The listing builds one solid part. Answer for the finished solid, in the listing's coordinates (mm). Face numbers are marked on the shaded views. A direction names the side the tool comes from. Give positions to 0.01 mm unless a question says otherwise; leave off trailing zeros. Order: outer loops, then holes, each group sorted by start corner. A loop starts at its lowest first (then second) coordinate and runs counter-clockwise, first axis right, second up. Notation, with made-up numbers: (60, -26.75) - (100, -26.75) arc R22 ccw to (100, -9.75) - close; hole circle Ø11 at (59.25, 74). An arc over 180 degrees is marked (long way). Use a Markdown table: item, result. Add a question column.
1) Find section C-C, the plane z = 1. Determine the outline of the cut face in (x, y), plus the area to 3 significant figures.
2) Straight lines are drawn through the part: line 1 (X direction, y = 18.25, z = -6.25); line 2 (Y direction, x = -21, z = 4.5); line 3 (Y direction, x = 14, z = 6.5). For each, find the intervals that lie inside material, in ascending order.
3) Find section D-D, the plane y = 2.25. Determine the outline of the cut face in (x, z).
4) Flat-ended cylindrical pins translate along their axes: pin 1 (5 mm diameter, centred on x = -20.5, z = 0.5, fed in from +Y); pin 2 (2 mm diameter, centred on x = 14.5, z = -3.5, fed in from +Y). Find the tip coordinate at first contact, or state that the pin passes through.
5) The mould has two halves that part along X. Classify the marked faces 1, 2 and 3: released by +X, released by -X, zero draft, split by the parting line, or undercut.
6) For the marked faces 4 and 5, determine the directions among +Z, -Z, +X, -X, +Y, -Y from which every point of the face is accessible in a straight line to the end or side of a thin tool.
7) Find section A-A, the plane y = 12.25. Determine the outline of the cut face in (x, z), plus the area to 3 significant figures.
8) Find section B-B, the plane x = -7. Determine the outline of the cut face in (y, z).
from build123d import *

# Parameters (mm, degrees)
SKETCH1_W           = 52
SKETCH1_H           = 18
BOSS_EXTRUDE1_DEPTH = 25.5
SKETCH2_W           = 46.1
SKETCH2_H           = 14.1
CUT_EXTRUDE1_DEPTH  = 2.5
SKETCH4_W           = 40
SKETCH4_H           = 18
CUT_EXTRUDE2_DEPTH  = 22.5
SKETCH5_W           = 25
SKETCH5_H           = 10
CUT_EXTRUDE3_DEPTH  = 4
FILLET1_R           = 2
FILLET2_R           = 2


with BuildPart() as part:
    # Sketch1 → Boss-Extrude1 (new body)
    with BuildSketch(Plane(origin=(0, 0, 0), x_dir=(1, 0, 0), z_dir=(0, 1, 0))):
        Rectangle(SKETCH1_W, SKETCH1_H)
    extrude(amount=BOSS_EXTRUDE1_DEPTH)

    # Sketch2 → Cut-Extrude1 (cut)
    with BuildSketch(Plane(origin=(0, 25.5, 0), x_dir=(1, 0, 0), z_dir=(0, 1, 0))):
        Rectangle(SKETCH2_W, SKETCH2_H)
    extrude(amount=-CUT_EXTRUDE1_DEPTH, mode=Mode.SUBTRACT)

    # Sketch4 → Cut-Extrude2 (cut)
    with BuildSketch(Plane(origin=(0, 25.5, 0), x_dir=(1, 0, 0), z_dir=(0, 1, 0))):
        Rectangle(SKETCH4_W, SKETCH4_H)
    extrude(amount=-CUT_EXTRUDE2_DEPTH, mode=Mode.SUBTRACT)

    # Sketch5 → Cut-Extrude3 (cut, through all)
    with BuildSketch(Plane(origin=(0, 3, 0), x_dir=(1, 0, 0), z_dir=(0, 1, 0))):
        Rectangle(SKETCH5_W, SKETCH5_H)
    extrude(amount=-CUT_EXTRUDE3_DEPTH, mode=Mode.SUBTRACT)

    # Fillet1
    fillet1_edges = [part.edges().sort_by_distance(p)[0] for p in [
        (-26, 12.75, -9),
        (26, 12.75, -9),
        (26, 12.75, 9),
        (-26, 12.75, 9),
    ]]
    fillet(fillet1_edges, radius=FILLET1_R)

    # Fillet2
    fillet2_edges = [part.edges().sort_by_distance(p)[0] for p in [
        (-12.5, 1.5, 5),
        (-12.5, 1.5, -5),
        (12.5, 1.5, -5),
        (12.5, 1.5, 5),
    ]]
    fillet(fillet2_edges, radius=FILLET2_R)


solid = part.part
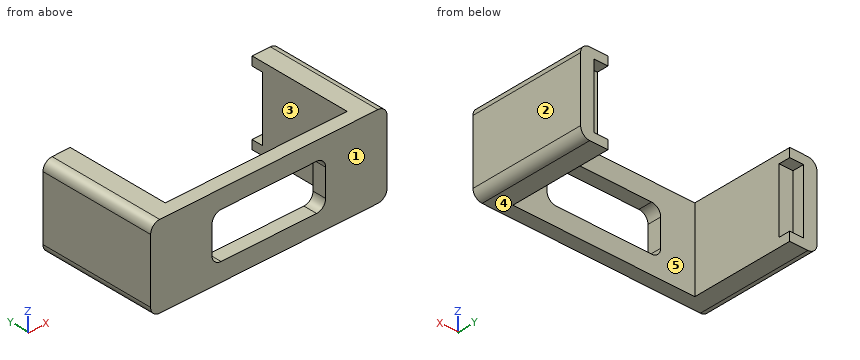
The answers:
| question | item | result |
|---|---|---|
| 1 | outline | (-26, 0) - (-12.5, 0) - (-12.5, 3) - (-20, 3) - (-20, 23) - (-23.05, 23) - (-23.05, 25.5) - (-26, 25.5) - close; (12.5, 0) - (26, 0) - (26, 25.5) - (23.05, 25.5) - (23.05, 23) - (20, 23) - (20, 3) - (12.5, 3) - close |
| 1 | area | 336 mm2 |
| 2 | line 1 | -26 to -20, 20 to 26 |
| 2 | line 2 | 0 to 23 |
| 2 | line 3 | 0 to 3 |
| 3 | outline | (-26, -7) arc R2 ccw to (-24, -9) - (24, -9) arc R2 ccw to (26, -7) - (26, 7) arc R2 ccw to (24, 9) - (-24, 9) arc R2 ccw to (-26, 7) - close; hole (-12.5, -3) arc R2 ccw to (-10.5, -5) - (10.5, -5) arc R2 ccw to (12.5, -3) - (12.5, 3) arc R2 ccw to (10.5, 5) - (-10.5, 5) arc R2 ccw to (-12.5, 3) - close |
| 4 | pin 1 | y = 23 |
| 4 | pin 2 | y = 3 |
| 5 | face 1 | zero draft |
| 5 | face 2 | released by +X |
| 5 | face 3 | undercut |
| 6 | face 4 | -Z, +X, -X, +Y, -Y |
| 6 | face 5 | +Z, -Z, +Y |
| 7 | outline | (-26, -7) arc R2 ccw to (-24, -9) - (-20, -9) - (-20, 9) - (-24, 9) arc R2 ccw to (-26, 7) - close; (20, -9) - (24, -9) arc R2 ccw to (26, -7) - (26, 7) arc R2 ccw to (24, 9) - (20, 9) - close |
| 7 | area | 213 mm2 |
| 8 | outline | (0, -9) - (3, -9) - (3, -5) - (0, -5) - close; (0, 5) - (3, 5) - (3, 9) - (0, 9) - close |
